from build123d import *

# Parameters (mm, degrees)
CROQUIS2_W              = 51.502836605
CROQUIS2_H              = 23.6
SALIENTE_EXTRUIR1_DEPTH = 11
CROQUIS4_W              = 2
CROQUIS4_H              = 5.8
SALIENTE_EXTRUIR2_DEPTH = 51.502837
CORTAR_EXTRUIR1_START   = -23.6
CORTAR_EXTRUIR1_DEPTH   = 23.6
CORTAR_EXTRUIR2_START   = -13
CROQUIS6_R              = 1.625
CORTAR_EXTRUIR2_DEPTH   = 13


with BuildPart() as part:
    # Croquis2 → Saliente-Extruir1 (new body)
    with BuildSketch(Plane.XY):
        with Locations((49.751418302, 20)):
            Rectangle(CROQUIS2_W, CROQUIS2_H)
    extrude(amount=SALIENTE_EXTRUIR1_DEPTH)

    # Croquis4 → Saliente-Extruir2 (add)
    with BuildSketch(Plane(origin=(75.502836605, 0, 0), x_dir=(0, 0, -1), z_dir=(1, 0, 0))):
        with Locations((-12, 11.1)):
            Rectangle(CROQUIS4_W, CROQUIS4_H)
        with Locations((-12, 28.9)):
            Rectangle(CROQUIS4_W, CROQUIS4_H)
    extrude(amount=-SALIENTE_EXTRUIR2_DEPTH)

    # Croquis5 → Cortar-Extruir1 (cut)
    with BuildSketch(Plane.XZ.offset(-8.2).offset(CORTAR_EXTRUIR1_START)):
        Polygon((49.751418302, 0), (34.751418302, 0), (34.751418302, 5), (49.751418302, 5), (64.751418302, 5), (64.751418302, 0), align=None)
    extrude(amount=CORTAR_EXTRUIR1_DEPTH, mode=Mode.SUBTRACT)

    # Croquis6 → Cortar-Extruir2 (cut)
    with BuildSketch(Plane.XY.offset(13).offset(CORTAR_EXTRUIR2_START)):
        with Locations((28.442619987, 11.1)):
            Circle(CROQUIS6_R)
        with Locations((28.442619987, 28.9)):
            Circle(CROQUIS6_R)
        with Locations((70.502836605, 11.1)):
            Circle(CROQUIS6_R)
        with Locations((70.502836605, 28.9)):
            Circle(CROQUIS6_R)
    extrude(amount=CORTAR_EXTRUIR2_DEPTH, mode=Mode.SUBTRACT)


solid = part.part
For this review, take the finished solid that the model builds, in its own axes (mm). A direction names the side the tool comes from. Round coordinates to 2 decimals unless told otherwise and drop trailing zeros. Write each loop counter-clockwise with the first axis right and the second up, starting at its lowest first coordinate (ties: lowest second). Pieces come first, ordered by that corner, then holes. Notation, with made-up numbers: (77, -21.5) -> (81, -21.5) arc R13 ccw to (81, -11.5) -> close; hole circle Ø4 at (-36.5, 36.25). An arc over 180 degrees is marked (long way). Put each result on its own line as item: value.
Q1. Consider section B-B on z = 8.5. State the section outline as (x, y) points (3 decimals), and give its area (3 significant figures).
Determined:
outline: (24, 8.2) -> (75.503, 8.2) -> (75.503, 31.8) -> (24, 31.8) -> close; hole circle Ø3.25 at (28.443, 11.1); hole circle Ø3.25 at (28.443, 28.9); hole circle Ø3.25 at (70.503, 11.1); hole circle Ø3.25 at (70.503, 28.9)
area: 1,180 mm^2
Q2. Machinability: for faces 4 (the flat face through (34.751, 20, 2)), 5 (the flat face through (29, 20, 0)), 6 (the flat face through (49, 20, 11)), which of the approach directions +Z, -Z, +X, -X, +Y, -Y give a long, thin tool a straight path to every point of the face, cutting with its end or side? Answer none if there is none.
Determined:
face 4: -Z, +Y, -Y
face 5: -Z, +X, -X, +Y, -Y
face 6: +Z, +X, -X
Q3. Consider section A-A on z = 4. State the section outline as (x, y) points (3 decimals).
Determined:
outline: (24, 8.2) -> (34.751, 8.2) -> (34.751, 31.8) -> (24, 31.8) -> close; (64.751, 8.2) -> (75.503, 8.2) -> (75.503, 31.8) -> (64.751, 31.8) -> close; hole circle Ø3.25 at (28.443, 11.1); hole circle Ø3.25 at (28.443, 28.9); hole circle Ø3.25 at (70.503, 11.1); hole circle Ø3.25 at (70.503, 28.9)
Q4. The part is to be moulded in two halves that separate along Y. For faces 1 (the cylindrical face through (68.88, 11.17, 6.41)), 2 (the flat face through (50, 20, 5)), 3 (the flat face through (50, 8.2, 8)), say which applies: released by +Y, released by -Y, zero draft, split by the parting line, or undercut.
Determined:
face 1: undercut
face 2: zero draft
face 3: released by -Y
Q5. Clearance check with flat-ended pins moving along their axes: pin 1 Ø2.5 at (x, y) = (70.5, 28.9) entering from +Z; pin 2 Ø1.5 at (x, y) = (33, 16) entering from +Z. State where each tip first meets the part, or that it passes through.
Determined:
pin 1: passes through
pin 2: stops at z = 11
Q6. Consider section C-C on y = 11.1. State the section outline as (x, z) points.
Determined:
outline: (24, 0) -> (26.82, 0) -> (26.82, 13) -> (24, 13) -> close; (30.07, 0) -> (34.75, 0) -> (34.75, 5) -> (64.75, 5) -> (64.75, 0) -> (68.88, 0) -> (68.88, 13) -> (30.07, 13) -> close; (72.13, 0) -> (75.5, 0) -> (75.5, 13) -> (72.13, 13) -> close
Q7. To check wall thickness, follow L1, parallel to X at y = 29, z = 3; L2, parallel to Y at x = 68.5, z = 12.75; L3, parallel to Y at x = 71, z = 12.25. State the ranges of each line that lie inside material, in increasing order. Write a range as [from, to].
Determined:
L1: x = [24, 26.82], [30.06, 34.75], [64.75, 68.88], [72.12, 75.5]
L2: y = [8.2, 14], [26, 31.8]
L3: y = [8.2, 9.55], [12.65, 14], [26, 27.35], [30.45, 31.8]
Q8. Consider section D-D on x = 36. State the section outline as (y, z) points, and give its area (3 significant figures).
Determined:
outline: (8.2, 5) -> (31.8, 5) -> (31.8, 13) -> (26, 13) -> (26, 11) -> (14, 11) -> (14, 13) -> (8.2, 13) -> close
area: 165 mm^2
